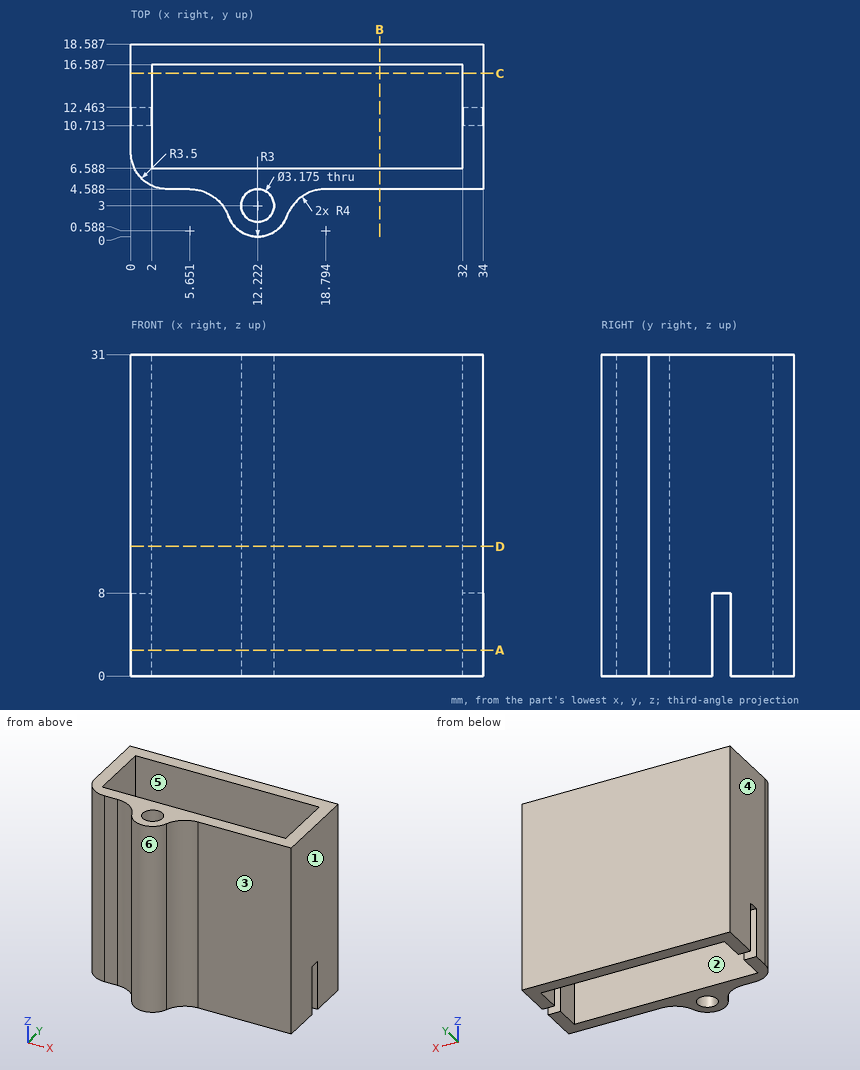
Design review of the part shown in the three views and the two pictorial views. Dimensions are in mm from the part's minimum x, y and z. A direction names the side the tool comes from. Round coordinates to 2 decimals unless told otherwise and drop trailing zeros. Write each loop counter-clockwise with the first axis right and the second up, starting at its lowest first coordinate (ties: lowest second). Pieces come first, ordered by that corner, then holes.
Item 1: Consider section A-A on z = 2.5. Give the boundary of the cut face in (x, y) (1 decimal).
Item 2: For the marked faces 1, 2 and 3, list the 3-axis set-ups (+Z, -Z, +X, -X, +Y, -Y) from which the entire face can be reached by the end or side of a thin tool; tool diameter is ignored.
Item 3: For pin 1 Ø10 at (x, z) = (22.5, 19) entering from -Y; pin 2 Ø1.5 at (x, y) = (20, 2) entering from -Z; pin 3 Ø7.5 at (x, z) = (28, 16) entering from -Y; pin 4 Ø0.5 at (x, y) = (1.5, 12) entering from -Z, all flat-tipped, find the tip position at first contact; note any pin that passes through.
Item 4: Consider section C-C on y = 15.75. Give the boundary of the cut face in (x, z).
Item 5: Wall thickness on L1, parallel to Y at x = 5, z = 19; L2, parallel to X at y = 13.25, z = 4; L3, parallel to X at y = 4.25, z = 15.5 (1 decimal): over which ranges is each line inside the solid? List them lowest first.
Item 6: Draft analysis for pull direction Y (two halves, no side actions). For the marked faces 4, 5 and 6, state which applies: released by +Y, released by -Y, zero draft, split by the parting line, or undercut.
Item 7: Consider section B-B on x = 24. Give the boundary of the cut face in (y, z), and give its area (3 significant figures).
Item 8: Consider section D-D on z = 12.5. Give the boundary of the cut face in (x, y) (1 decimal).
Check values:
1. outline: (0, 8.1) arc R3.5 ccw to (3.5, 4.6) - (5.7, 4.6) arc R4 cw to (9.4, 2) arc R3 ccw to (15, 2) arc R4 cw to (18.8, 4.6) - (34, 4.6) - (34, 10.7) - (32, 10.7) - (32, 6.6) - (2, 6.6) - (2, 10.7) - (0, 10.7) - close; (0, 12.5) - (2, 12.5) - (2, 16.6) - (32, 16.6) - (32, 12.5) - (34, 12.5) - (34, 18.6) - (0, 18.6) - close; hole circle Ø3.2 at (12.2, 3)
2. face 1: +Z, -Z, +X, +Y, -Y
2. face 2: +Z, -Z
2. face 3: +Z, -Z, +X, -Y
3. pin 1: stops at y = 4.37
3. pin 2: passes through
3. pin 3: stops at y = 4.59
3. pin 4: stops at z = 8
4. outline: (0, 0) - (2, 0) - (2, 31) - (0, 31) - close; (32, 0) - (34, 0) - (34, 31) - (32, 31) - close
5. L1: y = 4.59 to 6.59, 16.59 to 18.59
5. L2: x = 0 to 2, 32 to 34
5. L3: x = 7.3 to 11.2, 13.2 to 17.2
6. face 4: zero draft
6. face 5: undercut
6. face 6: released by -Y
7. outline: (4.59, 0) - (6.59, 0) - (6.59, 31) - (4.59, 31) - close; (16.59, 0) - (18.59, 0) - (18.59, 31) - (16.59, 31) - close
7. area: 124 mm2
8. outline: (0, 8.1) arc R3.5 ccw to (3.5, 4.6) - (5.7, 4.6) arc R4 cw to (9.4, 2) arc R3 ccw to (15, 2) arc R4 cw to (18.8, 4.6) - (34, 4.6) - (34, 18.6) - (0, 18.6) - close; hole (2, 6.6) - (32, 6.6) - (32, 16.6) - (2, 16.6) - close; hole circle Ø3.2 at (12.2, 3)
